Model file for the job. Use its own axes, mm. A direction names the side the tool comes from. Coordinates: 2 decimals unless noted, no trailing zeros. Write each loop counter-clockwise with the first axis right and the second up, starting at its lowest first coordinate (ties: lowest second). Pieces come first, ordered by that corner, then holes. Notation, with made-up numbers: (-27.5, 35.25) - (-6.5, 35.25) arc R7 cw to (-6.5, 40.25) - close; hole circle Ø10 at (46.25, 59). An arc over 180 degrees is marked (long way). Put each result on its own line as item: value. Start each with the question number.
1. Pull direction Y, two halves, no side cores. Call faces 4 (the face through (47.5, 0, 26)), 5 (the face through (-1, -30, 15)), 6 (the face through (49.5, 0, 15)): released by +Y, released by -Y, zero draft, split by the parting line, or undercut.
2. Saw through at B-B, the plane x = 12. Write the cut outline in (y, z).
3. Saw through at A-A, the plane z = 9.5. Write the cut outline in (x, y), plus the area to 3 significant figures.
4. Drill centre lines: L1, parallel to Y at x = -31, z = 3.5; L2, parallel to X at y = -12, z = 21.5; L3, parallel to X at y = 24, z = 19.75. Where is each one in solid material? Low to high. Write a range as from..to.
5. Saw through at C-C, the plane y = -2. Write the cut outline in (x, z), plus the area to 3 significant figures.
6. Which spindle directions (+Z, -Z, +X, -X, +Y, -Y) get a long thin tool onto all of the face, cutting with end or side? Do faces 1 (the face through (-1, 30, 15)), 2 (the face through (-47.5, 0, 26)), 3 (the face through (-47, 0, 19)). Say none if no direction does.
7. Drop a flat-ended pin along its axis: P1, Ø0.8, axis at x = 46.5, y = 6.5, coming from the +Z side. Give the stop position or say it passes through.
```python
from build123d import *

# Parameters (mm, degrees)
SKETCH003_W     = 99
SKETCH003_H     = 60
PAD002_DEPTH    = 30
SKETCH004_W     = 95
SKETCH004_H     = 56
POCKET001_DEPTH = 27
PAD003_DEPTH    = 0.5
PAD004_DEPTH    = 0.5
SKETCH007_W     = 56
SKETCH007_H     = 2
PAD005_DEPTH    = 1.5
SKETCH008_W     = 56
SKETCH008_H     = 2
PAD006_DEPTH    = 1.5
FILLET_R        = 1
FILLET001_R     = 0.45


with BuildPart() as part:
    # Sketch003 → Pad002 (new body)
    with BuildSketch(Plane.XY):
        Rectangle(SKETCH003_W, SKETCH003_H)
    extrude(amount=PAD002_DEPTH)

    # Sketch004 (on Face6 of Pad002) → Pocket001 (cut)
    with BuildSketch(Plane.XY.offset(30)):
        Rectangle(SKETCH004_W, SKETCH004_H)
    extrude(amount=-POCKET001_DEPTH, mode=Mode.SUBTRACT)

    # Sketch005 (on Face8 of Pocket001) → Pad003 (join)
    with BuildSketch(Plane.XZ.offset(-28)):
        with BuildLine():
            ThreePointArc((-37.5, 28), (-38.3, 27.2), (-37.5, 26.4))
            Line((-37.5, 26.4), (-33, 26.4))
            ThreePointArc((-33, 26.4), (-32.2, 27.2), (-33, 28))
            Line((-37.5, 28), (-33, 28))
        make_face()
        with BuildLine():
            ThreePointArc((33, 28), (32.2, 27.2), (33, 26.4))
            Line((33, 26.4), (37.5, 26.4))
            ThreePointArc((37.5, 26.4), (38.3, 27.2), (37.5, 28))
            Line((33, 28), (37.5, 28))
        make_face()
    extrude(amount=PAD003_DEPTH)

    # Sketch006 (on Face10 of Pad003) → Pad004 (join)
    with BuildSketch(Plane(origin=(0, -28, 0), x_dir=(-1, 0, 0), z_dir=(0, 1, 0))):
        with BuildLine():
            ThreePointArc((-37.5, 28), (-38.3, 27.2), (-37.5, 26.4))
            Line((-37.5, 26.4), (-33, 26.4))
            ThreePointArc((-33, 26.4), (-32.2, 27.2), (-33, 28))
            Line((-37.5, 28), (-33, 28))
        make_face()
        with BuildLine():
            ThreePointArc((33, 28), (32.2, 27.2), (33, 26.4))
            Line((33, 26.4), (37.5, 26.4))
            ThreePointArc((37.5, 26.4), (38.3, 27.2), (37.5, 28))
            Line((33, 28), (37.5, 28))
        make_face()
    extrude(amount=PAD004_DEPTH)

    # Sketch007 (on Face7 of Pad004) → Pad005 (join)
    with BuildSketch(Plane(origin=(47.5, 0, 0), x_dir=(0, -1, 0), z_dir=(-1, 0, 0))):
        with Locations((0, 20)):
            Rectangle(SKETCH007_W, SKETCH007_H)
    extrude(amount=PAD005_DEPTH)

    # Sketch008 (on Face9 of Pad005) → Pad006 (join)
    with BuildSketch(Plane.YZ.offset(-47.5)):
        with Locations((0, 20)):
            Rectangle(SKETCH008_W, SKETCH008_H)
    extrude(amount=PAD006_DEPTH)

    # Fillet
    fillet_edges = [part.edges().sort_by_distance(p)[0] for p in [
        (-46, 28, 20),
        (-46, -28, 20),
        (46, 28, 20),
        (46, -28, 20),
    ]]
    fillet(fillet_edges, radius=FILLET_R)

    # Fillet001
    fillet001_edges = [part.edges().sort_by_distance(p)[0] for p in [
        (-38.3, 27.5, 27.2),
        (-35.25, 27.5, 26.4),
        (-32.2, 27.5, 27.2),
        (-35.25, 27.5, 28),
        (32.2, 27.5, 27.2),
        (35.25, 27.5, 26.4),
        (38.3, 27.5, 27.2),
        (35.25, 27.5, 28),
        (38.3, -27.5, 27.2),
        (35.25, -27.5, 26.4),
        (32.2, -27.5, 27.2),
        (35.25, -27.5, 28),
        (-32.2, -27.5, 27.2),
        (-35.25, -27.5, 26.4),
        (-38.3, -27.5, 27.2),
        (-35.25, -27.5, 28),
    ]]
    fillet(fillet001_edges, radius=FILLET001_R)


solid = part.part
```
Final values:
1. face 4: undercut
1. face 5: released by -Y
1. face 6: zero draft
2. outline: (-30, 0) - (30, 0) - (30, 30) - (28, 30) - (28, 3) - (-28, 3) - (-28, 30) - (-30, 30) - close
3. outline: (-49.5, -30) - (49.5, -30) - (49.5, 30) - (-49.5, 30) - close; hole (-47.5, -28) - (47.5, -28) - (47.5, 28) - (-47.5, 28) - close
3. area: 620 mm²
4. L1: y = -30..-28, 28..30
4. L2: x = -49.5..-47.5, 47.5..49.5
4. L3: x = -49.5..-46, 46..49.5
5. outline: (-49.5, 0) - (49.5, 0) - (49.5, 30) - (47.5, 30) - (47.5, 21) - (46, 21) - (46, 19) - (47.5, 19) - (47.5, 3) - (-47.5, 3) - (-47.5, 19) - (-46, 19) - (-46, 21) - (-47.5, 21) - (-47.5, 30) - (-49.5, 30) - close
5. area: 411 mm²
6. face 1: +Z, -Z, +X, -X, +Y
6. face 2: +Z
6. face 3: none
7. P1: stops at z = 21
